Can you work these out from the model? Positions are in its coordinate system, mm. Give positions to 0.01 mm unless a question says otherwise; leave off trailing zeros. Loops run counter-clockwise (first coordinate to the right, second up) from the corner with the lowest first, then second, coordinate; pieces in that order, holes last. Notation, with made-up numbers: (-38, -36) - (20, -36) arc R19 cw to (20, -13) - close; hole circle Ø8 at (73, 38). An arc over 180 degrees is marked (long way). Answer as a JSON object with one key per item and string values. Group by question number.
Item 1: Please list where these lines run through material, in increasing order: L1, parallel to X at y = 5.25, z = 225; L2, parallel to X at y = 3.5, z = 225; L3, parallel to Y at x = 4.75, z = 665.
Item 2: Will these pins go through, and if not, where does the flat tip stop? pin 1 (2.5 mm diameter, centred on x = 0, z = 785, fed in from +Y); pin 2 (0.6 mm diameter, centred on y = 6, z = 290, fed in from +X); pin 3 (5 mm diameter, centred on x = -0.5, z = 154, fed in from -Y); pin 4 (3 mm diameter, centred on x = 6, z = 471.5, fed in from +Y).
Item 3: Suppose I cut it at A-A on z = 849. Write out the boundary of the cut face in (x, y), and give its area (3 significant figures).
from build123d import *

# Parameters (mm, degrees)
BOSS_EXTRUDE1_DEPTH = 1100
SKETCH2_R           = 1.5
CUT_EXTRUDE1_DEPTH  = 1101.043608227


with BuildPart() as part:
    # Sketch1 → Boss-Extrude1 (new body)
    with BuildSketch(Plane.XY):
        Polygon((3.9, 0), (-3.9, 0), (-7.5, 5.5), (-3.9, 5.5), (-3.9, 6.3), (3.9, 6.3), (3.9, 5.5), (7.5, 5.5), align=None)
    extrude(amount=BOSS_EXTRUDE1_DEPTH)

    # Sketch2 → Cut-Extrude1 (cut, through all)
    with BuildSketch(Plane(origin=(0, 6.3, 0), x_dir=(1, 0, 0), z_dir=(0, 1, 0))):
        with Locations(Location((0, -65, 0), (0, 0, 270))):
            Circle(SKETCH2_R)
        with Locations(Location((0, -145, 0), (0, 0, 270))):
            Circle(SKETCH2_R)
        with Locations(Location((0, -225, 0), (0, 0, 270))):
            Circle(SKETCH2_R)
        with Locations(Location((0, -305, 0), (0, 0, 270))):
            Circle(SKETCH2_R)
        with Locations(Location((0, -385, 0), (0, 0, 270))):
            Circle(SKETCH2_R)
        with Locations(Location((0, -465, 0), (0, 0, 270))):
            Circle(SKETCH2_R)
        with Locations(Location((0, -545, 0), (0, 0, 270))):
            Circle(SKETCH2_R)
        with Locations(Location((0, -625, 0), (0, 0, 270))):
            Circle(SKETCH2_R)
        with Locations(Location((0, -705, 0), (0, 0, 270))):
            Circle(SKETCH2_R)
        with Locations(Location((0, -785, 0), (0, 0, 270))):
            Circle(SKETCH2_R)
        with Locations(Location((0, -865, 0), (0, 0, 270))):
            Circle(SKETCH2_R)
        with Locations(Location((0, -945, 0), (0, 0, 270))):
            Circle(SKETCH2_R)
        with Locations(Location((0, -1025, 0), (0, 0, 270))):
            Circle(SKETCH2_R)
    extrude(amount=-CUT_EXTRUDE1_DEPTH, mode=Mode.SUBTRACT)


solid = part.part
Worked out:
{
 "1": {"L1": "x = -7.34 to -1.5, 1.5 to 7.34", "L2": "x = -6.19 to -1.5, 1.5 to 6.19", "L3": "y = 1.3 to 5.5"},
 "2": {"pin 1": "passes through", "pin 2": "stops at x = 3.9", "pin 3": "stops at y = 0", "pin 4": "stops at y = 5.5"},
 "3": {"outline": "(-7.5, 5.5) - (-3.9, 0) - (3.9, 0) - (7.5, 5.5) - (3.9, 5.5) - (3.9, 6.3) - (-3.9, 6.3) - (-3.9, 5.5) - close", "area": "68.9 mm2"}
}
